```python
from build123d import *
from build123d.topology import SkipClean

# Parameters (mm, degrees)
CUT_EXTRUDE1_DEPTH      = 57.00892786
CUT_EXTRUDE1_DEPTH_BACK = 57.00892786
CUT_EXTRUDE2_DEPTH      = 81.024996095
CUT_EXTRUDE2_DEPTH_BACK = 81.024996095
SKETCH2_R               = 16


with BuildPart() as part:
    # Sketch1 → Revolve8 (revolve)
    with SkipClean():  # the faces are left unmerged after this step: merging them gives an invalid solid
        with BuildSketch(Plane(origin=(0, 0, 0), x_dir=(1, 0, 0), z_dir=(0, 1, 0)), mode=Mode.PRIVATE) as revolve8_sk:
            Polygon((-33, 0), (-24, 0), (-24, 24), (-24, 32), (-33, 32), align=None)
            Polygon((-24, 0), (-14, 0), (-14, 22), (-14, 24), (-24, 24), align=None)
            with BuildLine():
                Line((-14, 22), (-14, 0))
                Line((-14, 0), (-4, 0))
                ThreePointArc((-4, 0), (-2.828427125, 2.828427125), (0, 4))
                Line((0, 4), (0, 22))
                Line((0, 22), (-14, 22))
            make_face()
            with BuildLine():
                ThreePointArc((-3, 0), (-2.121320344, -2.121320344), (0, -3))
                Line((0, -3), (0, 0))
                Line((0, 0), (-3, 0))
            make_face()
            with BuildLine():
                Line((0, 0), (0, -3))
                ThreePointArc((0, -3), (2.121320344, -2.121320344), (3, 0))
                Line((3, 0), (0, 0))
            make_face()
            with BuildLine():
                Line((0, 0), (3, 0))
                ThreePointArc((3, 0), (2.121320344, 2.121320344), (0, 3))
                Line((0, 3), (0, 0))
            make_face()
            with BuildLine():
                Line((-3, 0), (0, 0))
                Line((0, 0), (0, 3))
                ThreePointArc((0, 3), (-2.121320344, 2.121320344), (-3, 0))
            make_face()
            with BuildLine():
                ThreePointArc((-4, 0), (-2.828427125, -2.828427125), (0, -4))
                Line((0, -4), (0, -3))
                ThreePointArc((0, -3), (-2.121320344, -2.121320344), (-3, 0))
                Line((-3, 0), (-4, 0))
            make_face()
            with BuildLine():
                Line((0, -3), (0, -4))
                ThreePointArc((0, -4), (2.828427125, -2.828427125), (4, 0))
                Line((4, 0), (3, 0))
                ThreePointArc((3, 0), (2.121320344, -2.121320344), (0, -3))
            make_face()
            with BuildLine():
                Line((3, 0), (4, 0))
                ThreePointArc((4, 0), (2.828427125, 2.828427125), (0, 4))
                Line((0, 4), (0, 3))
                ThreePointArc((0, 3), (2.121320344, 2.121320344), (3, 0))
            make_face()
            with BuildLine():
                ThreePointArc((0, 4), (-2.828427125, 2.828427125), (-4, 0))
                Line((-4, 0), (-3, 0))
                ThreePointArc((-3, 0), (-2.121320344, 2.121320344), (0, 3))
                Line((0, 3), (0, 4))
            make_face()
            with BuildLine():
                Line((4, 0), (14, 0))
                Line((14, 0), (14, 22))
                Line((14, 22), (0, 22))
                Line((0, 22), (0, 4))
                ThreePointArc((0, 4), (2.828427125, 2.828427125), (4, 0))
            make_face()
            Polygon((14, 0), (24, 0), (24, 24), (14, 24), (14, 22), align=None)
            Polygon((24, 24), (24, 0), (33, 0), (33, 32), (24, 32), align=None)
        revolve(revolve8_sk.sketch.rotate(Axis((-33, 0, 0), (1, 0, 0)), 180), axis=Axis((-33, 0, 0), (1, 0, 0)))

    # Sketch1_4 → Cut-Extrude1 (cut, two sides: drawn at the far end of the back side and taken through both)
    with BuildSketch(Plane(origin=(0, 0, 0), x_dir=(1, 0, 0), z_dir=(0, 1, 0)).offset(-CUT_EXTRUDE1_DEPTH_BACK)):
        with BuildLine():
            ThreePointArc((-3, 0), (-2.121320344, -2.121320344), (0, -3))
            Line((0, -3), (0, 0))
            Line((0, 0), (-3, 0))
        make_face()
        with BuildLine():
            Line((0, 0), (0, -3))
            ThreePointArc((0, -3), (2.121320344, -2.121320344), (3, 0))
            Line((3, 0), (0, 0))
        make_face()
        with BuildLine():
            Line((0, 0), (3, 0))
            ThreePointArc((3, 0), (2.121320344, 2.121320344), (0, 3))
            Line((0, 3), (0, 0))
        make_face()
        with BuildLine():
            Line((-3, 0), (0, 0))
            Line((0, 0), (0, 3))
            ThreePointArc((0, 3), (-2.121320344, 2.121320344), (-3, 0))
        make_face()
    extrude(amount=CUT_EXTRUDE1_DEPTH + CUT_EXTRUDE1_DEPTH_BACK, mode=Mode.SUBTRACT)

    # Sketch2 → Cut-Extrude2 (cut, two sides: drawn at the far end of the back side and taken through both)
    with BuildSketch(Plane(origin=(33, 0, 0), x_dir=(0, 0, -1), z_dir=(1, 0, 0)).offset(-CUT_EXTRUDE2_DEPTH_BACK)):
        Circle(SKETCH2_R)
    extrude(amount=CUT_EXTRUDE2_DEPTH + CUT_EXTRUDE2_DEPTH_BACK, mode=Mode.SUBTRACT)


solid = part.part
```
Can you work these out from the model? Positions are in its coordinate system, mm. A direction names the side the tool comes from. Coordinates: 2 decimals unless noted, no trailing zeros. Loops run counter-clockwise (first coordinate to the right, second up) from the corner with the lowest first, then second, coordinate; pieces in that order, holes last.
Item 1: Suppose I cut it at D-D (x = -16). Please give me the cut outline in (y, z), then the cut area to 3 significant figures.
Answers below:
outline: circle Ø48 at (0, 0); hole circle Ø32 at (0, 0)
area: 1,010 mm2
Item 2: Suppose I cut it at B-B (z = -12). Please give me the cut outline in (x, y).
Answers below:
outline: (-33, -29.66) - (-24, -29.66) - (-24, -20.78) - (-14, -20.78) - (-14, -18.44) - (14, -18.44) - (14, -20.78) - (24, -20.78) - (24, -29.66) - (33, -29.66) - (33, -10.58) - (-33, -10.58) - close; (-33, 10.58) - (33, 10.58) - (33, 29.66) - (24, 29.66) - (24, 20.78) - (14, 20.78) - (14, 18.44) - (-14, 18.44) - (-14, 20.78) - (-24, 20.78) - (-24, 29.66) - (-33, 29.66) - close
Item 3: Please list where these lines run through material, in increasing order: L1, parallel to Y at x = -16.5, z = 0; L2, parallel to Y at x = -8, z = 0; L3, parallel to X at y = 28, z = 10.
Answers below:
L1: y = -24 to -16, 16 to 24
L2: y = -22 to -16, 16 to 22
L3: x = -33 to -24, 24 to 33
Item 4: If we mould it in two halves opening along Z, with no side actions, what happens to faces 1 (the face through (18.93, -7.21, 22.89)), 2 (the face through (33, -15, -7)), 3 (the face through (-0.46, -15.62, 3.47))? For each: released by +Z, released by -Z, zero draft, split by the parting line, or undercut.
Answers below:
face 1: split by the parting line
face 2: zero draft
face 3: undercut
Item 5: Suppose I cut it at C-C (y = 18.5). Please give me the cut outline in (x, z).
Answers below:
outline: (-33, -26.11) - (-24, -26.11) - (-24, -15.29) - (-14, -15.29) - (-14, -11.91) - (14, -11.91) - (14, -15.29) - (24, -15.29) - (24, -26.11) - (33, -26.11) - (33, 26.11) - (24, 26.11) - (24, 15.29) - (14, 15.29) - (14, 11.91) - (-14, 11.91) - (-14, 15.29) - (-24, 15.29) - (-24, 26.11) - (-33, 26.11) - close; hole circle Ø6 at (0, 0)
Item 6: I'm going to push flat-ended pins straight in: pin 1 (1.5 mm diameter, centred on x = 21, z = 17, fed in from +Y); pin 2 (19 mm diameter, centred on y = 6.5, z = -10.5, fed in from -X); pin 3 (10 mm diameter, centred on x = -12.5, y = -14, fed in from -Z); pin 4 (1.5 mm diameter, centred on x = -4, z = 10.5, fed in from -Y). Where does each tip first touch, or does it pass through?
Answers below:
pin 1: stops at y = 17.66
pin 2: stops at x = -33
pin 3: stops at z = -22.15
pin 4: stops at y = -19.72
Item 7: Suppose I cut it at A-A (y = 0). Please give me the cut outline in (x, z).
Answers below:
outline: (-33, -32) - (-24, -32) - (-24, -24) - (-14, -24) - (-14, -22) - (14, -22) - (14, -24) - (24, -24) - (24, -32) - (33, -32) - (33, -16) - (-33, -16) - close; (-33, 16) - (33, 16) - (33, 32) - (24, 32) - (24, 24) - (14, 24) - (14, 22) - (-14, 22) - (-14, 24) - (-24, 24) - (-24, 32) - (-33, 32) - close
Item 8: Which directions (+Z, -Z, +X, -X, +Y, -Y) give clear straight access to the entire face, cutting with the end or side of a thin tool? Please do faces 4 (the face through (-14, 7, -21.2)), 5 (the face through (-33, 7, -15)).
Answers below:
face 4: none
face 5: +Z, -Z, -X, +Y, -Y
